Model file for the job. Use its own axes, mm. A direction names the side the tool comes from. Round coordinates to 2 decimals unless told otherwise and drop trailing zeros. Order: outer loops, then holes, each group sorted by start corner. A loop starts at its lowest first (then second) coordinate and runs counter-clockwise, first axis right, second up. Notation, with made-up numbers: M 16.25,-11.75 L 37.25,-11.75 A14 ccw 37.25,15.25 Z; hole C -11.75,-34.75 d5. An arc over 180 degrees is marked long. Return JSON: item names as keys, results as strings. Group by question number.
Item 1: Slice it at C-C on y = 20.5. Write the cut outline in (x, z).
Item 2: Which spindle directions (+Z, -Z, +X, -X, +Y, -Y) get a long thin tool onto all of the face, cutting with end or side? Do faces 4 (the face through (-15, 30, 0)), 5 (the face through (-11, 15, 0)). Say none if no direction does.
Item 3: Slice it at A-A on z = -0.3. Write the cut outline in (x, y).
Item 4: Pull direction X, two halves, no side cores. Call faces 1 (the face through (0, 30, 0)), 2 (the face through (9, 23, 0)), 3 (the face through (47.67, 16.37, -0.03)): pulls with the +X half, pulls with the -X half, needs draft (parallel to the pull), parting line crosses it, or undercut.
Item 5: Slice it at D-D on x = -11. Write the cut outline in (y, z), then the cut area to 3 significant figures.
Item 6: Pin check, flat tips, straight feed: pin 1 Ø1.5 at (y, z) = (20.5, -1.5) entering from -X; pin 2 Ø1.2 at (y, z) = (24.5, -1) entering from -X; pin 3 Ø1 at (y, z) = (22, 0.5) entering from +X. Stop position of each tip, or through.
Item 7: Slice it at B-B on y = 26.5. Write the cut outline in (x, z).
Item 8: Probe line 1 along X through (y, z) = (22.5, -1.15); line 2 along X through (y, z) = (25, -0.75); line 3 along Y through (x, z) = (10, -1.45). List the from-to ranges inside material, lowest first.
Autodesk Inventor part; units mm, degrees
ref_plane "YZ Plane" through (0, 0, 0) normal (1, 0, 0) x (0, 1, 0)
ref_plane "XZ Plane" through (0, 0, 0) normal (0, 1, 0) x (-1, 0, 0)
ref_plane "XY Plane" through (0, 0, 0) normal (0, 0, 1) x (1, 0, 0)
sketch "Náčrt1" plane through (0, 0, 0) normal (0, 0, 1) x (1, 0, 0)
  line L0 (0, 0) -> (0, 30)
  line L1 (0, 30) -> (-9, 30)
  line L2 (-9, 30) -> (-9, 15)
  line L3 (-9, 15) -> (-13, 15)
  line L4 (-13, 15) -> (-13, 30)
  line L5 (-13, 30) -> (-16.5756, 30)
  line L6 (-17.3878, 29.8276) -> (-78.8123, 2.5279)
  line L7 (-80, 0.7003) -> (-80, 0)
  line L8 (-80, 0) -> (0, 0)
  arc A0 (-78.8123, 2.5279) -> (-80, 0.7003) centre (-78, 0.7003) ccw
  arc A1 (-16.5756, 30) -> (-17.3878, 29.8276) centre (-16.5756, 28) ccw
  line L9 (0, 30) -> (9, 30)
  line L10 (9, 30) -> (9, 15)
  line L11 (9, 15) -> (13, 15)
  line L12 (13, 15) -> (13, 30)
  line L13 (13, 30) -> (16.5756, 30)
  line L14 (17.3878, 29.8276) -> (78.8123, 2.5279)
  line L15 (80, 0.7003) -> (80, 0)
  line L16 (80, 0) -> (0, 0)
  arc A2 (80, 0.7003) -> (78.8123, 2.5279) centre (78, 0.7003) ccw
  arc A3 (17.3878, 29.8276) -> (16.5756, 30) centre (16.5756, 28) ccw
  point P0 (-17, 30)
  point P1 (-80, 2)
  point P2 (17, 30)
  point P3 (80, 2)
  dimension "d0" = 15
  dimension "d1" = 15
  dimension "d4" = 4
  dimension "d5" = 4
  dimension "d6" = 9
  dimension "d7" = 2
  dimension "d8" = 80
  dimension "d9" = 2
extrude "Vysunutí1" add sketch "Náčrt1" along normal mid plane 4
equation "\"d10\" = d4"
properties part number "Leg"
Output values:
{
 "1": {"outline": "M -38.37,-2 L -13,-2 L -13,2 L -38.37,2 Z; M -9,-2 L 9,-2 L 9,2 L -9,2 Z; M 13,-2 L 38.37,-2 L 38.37,2 L 13,2 Z"},
 "2": {"face 4": "+Z, -Z, +X, -X, +Y", "face 5": "+Z, -Z, +Y"},
 "3": {"outline": "M -80,0 L 80,0 L 80,0.7 A2 ccw 78.81,2.53 L 17.39,29.83 A2 ccw 16.58,30 L 13,30 L 13,15 L 9,15 L 9,30 L -9,30 L -9,15 L -13,15 L -13,30 L -16.58,30 A2 ccw -17.39,29.83 L -78.81,2.53 A2 ccw -80,0.7 Z"},
 "4": {"face 1": "needs draft", "face 2": "undercut", "face 3": "pulls with the +X half"},
 "5": {"outline": "M 0,-2 L 15,-2 L 15,2 L 0,2 Z", "area": "60.0 mm²"},
 "6": {"pin 1": "x = -40.06", "pin 2": "x = -30.72", "pin 3": "x = 36.12"},
 "7": {"outline": "M -24.87,-2 L -13,-2 L -13,2 L -24.87,2 Z; M -9,-2 L 9,-2 L 9,2 L -9,2 Z; M 13,-2 L 24.87,-2 L 24.87,2 L 13,2 Z"},
 "8": {"line 1": "-33.87 to -13, -9 to 9, 13 to 33.87", "line 2": "-28.25 to -13, -9 to 9, 13 to 28.25", "line 3": "0 to 15"}
}
